from build123d import *

# Parameters (mm, degrees)
BODY_DEPTH                 = 15.875
SKETCH2_R                  = 12.7254
F_1_002_HOLE_DEPTH         = 333.466619565
SKETCH3_R                  = 3.96748
F_3124_HOLE_DEPTH          = 333.466619565
SLOT_DEPTH                 = 25.4
ANGULAR_CLEARANCE_DEPTH    = 8.9408
SKETCH6_R                  = 2.3749
PIN_HOLE_DEPTH             = 25.4
F_5_16_18_TAPPED_HOLE1_D   = 6.5278
F_1_4_20_TAPPED_HOLE1_D    = 5.1054
F_8_32_TAPPED_HOLE1_REACH  = 334.421
F_8_32_TAPPED_HOLE1_BORE_R = 1.7272


with BuildPart() as part:
    # Sketch1 → BODY (new, symmetric)
    with BuildSketch(Plane(origin=(0, 0, 0), x_dir=(0, 0, -1), z_dir=(1, 0, 0))):
        with BuildLine():
            Line((0, 22.225), (282.575, 22.225))
            Line((282.575, 22.225), (323.58444924, 9.069770125))
            ThreePointArc((323.58444924, 9.069770125), (330.112821091, -1.285751941), (321.052227723, -9.517527213))
            Line((321.052227723, -9.517527213), (0.88019802, -22.207563496))
            ThreePointArc((0.88019802, -22.207563496), (-22.220640447, -0.440185355), (0, 22.225))
        make_face()
    extrude(amount=BODY_DEPTH, both=True)

    # Sketch2 → 1.002 HOLE (cut, through all)
    with BuildSketch(Plane(origin=(15.875, 0, 0), x_dir=(0, 0, -1), z_dir=(1, 0, 0))):
        Circle(SKETCH2_R)
    extrude(amount=-F_1_002_HOLE_DEPTH, mode=Mode.SUBTRACT)

    # Sketch3 → .3124 HOLE (cut, through all)
    with BuildSketch(Plane(origin=(15.875, 0, 0), x_dir=(0, 0, -1), z_dir=(1, 0, 0))):
        with Locations((320.675, 0)):
            Circle(SKETCH3_R)
    extrude(amount=-F_3124_HOLE_DEPTH, mode=Mode.SUBTRACT)

    # Sketch4 → SLOT (cut, symmetric)
    with BuildSketch(Plane(origin=(0, 0, 0), x_dir=(1, 0, 0), z_dir=(0, 1, 0))):
        with BuildLine():
            Line((-8.9408, 336.55), (8.9408, 336.55))
            Line((8.9408, 336.55), (8.9408, 260.35))
            ThreePointArc((8.9408, 260.35), (8.01086403, 258.10493597), (5.7658, 257.175))
            Line((5.7658, 257.175), (-5.7658, 257.175))
            ThreePointArc((-5.7658, 257.175), (-8.01086403, 258.10493597), (-8.9408, 260.35))
            Line((-8.9408, 260.35), (-8.9408, 336.55))
        make_face()
    extrude(amount=SLOT_DEPTH, both=True, mode=Mode.SUBTRACT)

    # Sketch5 → ANGULAR CLEARANCE (cut, symmetric)
    with BuildSketch(Plane(origin=(0, 0, 0), x_dir=(0, 0, -1), z_dir=(1, 0, 0))):
        Polygon((263.525, -2.529744374), (234.95, -12.930193819), (263.525, -11.797622097), align=None)
    extrude(amount=ANGULAR_CLEARANCE_DEPTH, both=True, mode=Mode.SUBTRACT)

    # Sketch6 → PIN HOLE (cut, symmetric)
    with BuildSketch(Plane(origin=(0, 0, 0), x_dir=(1, 0, 0), z_dir=(0, 1, 0))):
        with Locations(Location((0, 0, 0), (0, 0, 270))):
            Circle(SKETCH6_R)
    extrude(amount=PIN_HOLE_DEPTH, both=True, mode=Mode.SUBTRACT)

    # 5/16-18 Tapped Hole1 (through all)
    with Locations(Plane(origin=(0, 22.225, 0), x_dir=(-1, 0, 0), z_dir=(0, 1, 0))):
        with Locations((0, -92.075)):
            Hole(F_5_16_18_TAPPED_HOLE1_D / 2)

    # 1/4-20 Tapped Hole1 (through all)
    with Locations(Plane(origin=(15.875, 0, 0), x_dir=(0, 0, -1), z_dir=(1, 0, 0))):
        with Locations((110.562035551, 11.171477956)):
            Hole(F_1_4_20_TAPPED_HOLE1_D / 2)

    # #8-32 Tapped Hole1 bore → #8-32 Tapped Hole1 (cut, up to next)
    with BuildSketch(Plane(origin=(0, -12.7, 0), x_dir=(-1, 0, 0), z_dir=(0, -1, 0)), mode=Mode.PRIVATE) as f_8_32_tapped_hole1_sk1:
        with Locations((12.3952, 320.675)):
            Circle(F_8_32_TAPPED_HOLE1_BORE_R)
    f_8_32_tapped_hole1_tool1 = extrude(f_8_32_tapped_hole1_sk1.sketch, amount=-F_8_32_TAPPED_HOLE1_REACH, mode=Mode.PRIVATE) & part.part
    add(f_8_32_tapped_hole1_tool1.solids().sort_by_distance((-12.3952, -12.7, -320.675))[0], mode=Mode.SUBTRACT)


solid = part.part
Can you work these out from the model? Positions are in its coordinate system, mm. A direction names the side the tool comes from. Round coordinates to 2 decimals unless told otherwise and drop trailing zeros. Order: outer loops, then holes, each group sorted by start corner. A loop starts at its lowest first (then second) coordinate and runs counter-clockwise, first axis right, second up. Notation, with made-up numbers: (11.5, 45) -> (49.5, 45) arc R4 ccw to (49.5, 49) -> close; hole circle Ø4 at (34, 50). An arc over 180 degrees is marked (long way). Write each question's results on one line, items separated by ' | '. Start each with the question number.
Item 1: Please list where these lines run through material, in increasing order: L1, parallel to Z at x = -13, y = -3.5; L2, parallel to X at y = 1.5, z = -306.5 (3 decimals); L3, parallel to Z at x = 6, y = -0.5.
Item 2: Which directions (+Z, -Z, +X, -X, +Y, -Y) give clear straight access to the entire face, cutting with the end or side of a thin tool? Please do faces 4 (the flat face through (0.13, -9.27, -245.01)), 5 (the flat face through (0.222, -15.774, -163.207)), 6 (the flat face through (0, 9, -257.175)).
Item 3: If we section it at A-A, the plane y = 0: Write out the boundary of the cut face in (x, z) (3 decimals).
Item 4: Thinking about a two-plate mould opening in Y: for faces 1 (the cylindrical face through (-12.359, 3.345, -322.808)), 2 (the cylindrical face through (0.222, -0.935, 22.205)), 3 (the flat face through (0, 22.225, -139)), which applies, +Y half, -Y half, draft (parallel to the pull), parting line (faces both ways), or undercut?
Item 5: If we section it at C-C, the plane z = -195: Write out the boundary of the cut face in (x, y) (3 decimals), then the cut area to 3 significant figures.
Item 6: If we section it at B-B, the plane z = -291: Write out the boundary of the cut face in (x, y) (3 decimals), then the cut area to 3 significant figures.
Item 7: Will these pins go through, and if not, where does the flat tip stop? pin 1 (4 mm diameter, centred on x = 0, z = -92.075, fed in from +Y) (3 decimals); pin 2 (12.5 mm diameter, centred on x = 1, y = 3.5, fed in from -Z); pin 3 (5 mm diameter, centred on x = 6, y = -6.5, fed in from -Z); pin 4 (4 mm diameter, centred on x = -12.4, z = -320.68, fed in from +Y).
Item 8: If we section it at D-D, the plane z = -136: Write out the boundary of the cut face in (x, y) (3 decimals), then the cut area to 3 significant figures.
Results:
1) L1: z = -329.53 to -322.54, -318.81 to -12.23, 12.23 to 21.95 | L2: x = -15.875 to -8.941, 8.941 to 15.875 | L3: z = -257.18 to -12.72, 12.72 to 22.22
2) face 4: -Z, -Y | face 5: -Z, +X, -X, -Y | face 6: -Z, +Y, -Y
3) outline: (-15.875, -330.2) -> (-8.941, -330.2) -> (-8.941, -324.642) -> (-15.875, -324.642) -> close; (-15.875, -316.708) -> (-8.941, -316.708) -> (-8.941, -260.35) arc R3.175 cw to (-5.766, -257.175) -> (5.766, -257.175) arc R3.175 cw to (8.941, -260.35) -> (8.941, -316.708) -> (15.875, -316.708) -> (15.875, -12.725) -> (-15.875, -12.725) -> close; (-15.875, 12.725) -> (15.875, 12.725) -> (15.875, 22.225) -> (-15.875, 22.225) -> close; (8.941, -330.2) -> (15.875, -330.2) -> (15.875, -324.642) -> (8.941, -324.642) -> close; hole circle Ø6.528 at (0, -92.075)
4) face 1: undercut | face 2: parting line | face 3: +Y half
5) outline: (-15.875, -14.514) -> (15.875, -14.514) -> (15.875, 22.225) -> (-15.875, 22.225) -> close | area: 1,170 mm2
6) outline: (-15.875, -10.709) -> (-8.941, -10.709) -> (-8.941, 19.522) -> (-15.875, 19.522) -> close; (8.941, -10.709) -> (15.875, -10.709) -> (15.875, 19.522) -> (8.941, 19.522) -> close | area: 419 mm2
7) pin 1: passes through | pin 2: stops at z = -257.54 | pin 3: stops at z = -257.79 | pin 4: stops at y = 10.64
8) outline: (-15.875, -16.852) -> (15.875, -16.852) -> (15.875, 22.225) -> (-15.875, 22.225) -> close | area: 1,240 mm2
